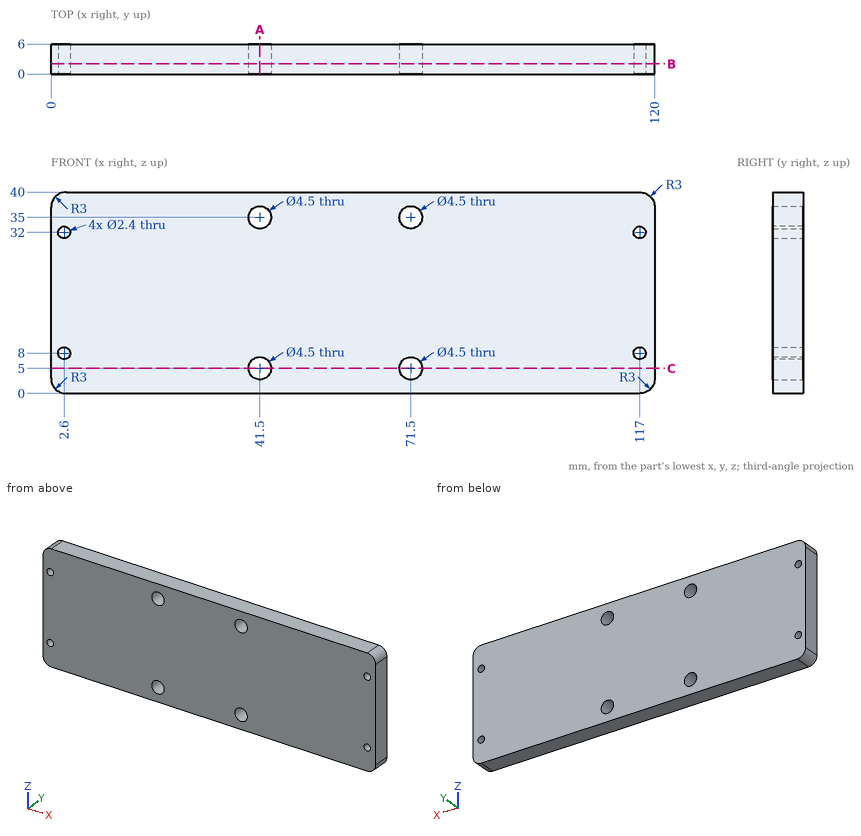
Geometry check sheet. Reference: drawing and pictorial views, mm from the part's lowest x, y, z. Give positions to 0.01 mm unless a question says otherwise; leave off trailing zeros. Loops run counter-clockwise (first coordinate to the right, second up) from the corner with the lowest first, then second, coordinate; pieces in that order, holes last. Notation, with made-up numbers: (48, 47) -> (57, 47) arc R20 ccw to (57, 54) -> close; hole circle Ø2 at (-26.75, 62.5). An arc over 180 degrees is marked (long way). Answer in a Markdown table with one row per item. Add a question column.
1) Cross-section at B-B on y = 2.05. State how many separate pieces and enclosed holes the cut face has, and give its area (3 significant figures).
2) Material ranges on probe 1 along X at (y, z) = (3.6, 35); probe 2 along X at (y, z) = (1.8, 32); probe 3 along Z at (x, y) = (71.5, 3.15), recorded low to high. Write a range as from..to.
3) Cross-section at C-C on z = 5. Record the boundary of the cut face in (x, y).
4) Cross-section at A-A on x = 41.5. Record the boundary of the cut face in (y, z), and give its area (3 significant figures).
Outcome:
| question | item | result |
|---|---|---|
| 1 | separate pieces | 1 |
| 1 | enclosed holes | 8 |
| 1 | area | 4,710 mm^2 |
| 2 | probe 1 | x = 0..39.25, 43.75..69.25, 73.75..120 |
| 2 | probe 2 | x = 0..1.4, 3.8..115.8, 118.2..120 |
| 2 | probe 3 | z = 0..2.75, 7.25..32.75, 37.25..40 |
| 3 | outline | (0, 0) -> (39.25, 0) -> (39.25, 6) -> (0, 6) -> close; (43.75, 0) -> (69.25, 0) -> (69.25, 6) -> (43.75, 6) -> close; (73.75, 0) -> (120, 0) -> (120, 6) -> (73.75, 6) -> close |
| 4 | outline | (0, 0) -> (6, 0) -> (6, 2.75) -> (0, 2.75) -> close; (0, 7.25) -> (6, 7.25) -> (6, 32.75) -> (0, 32.75) -> close; (0, 37.25) -> (6, 37.25) -> (6, 40) -> (0, 40) -> close |
| 4 | area | 186 mm^2 |
